Geometry check sheet. Reference: drawing and pictorial views, mm from the part's lowest x, y, z. A direction names the side the tool comes from. Round coordinates to 2 decimals unless told otherwise and drop trailing zeros. Order: outer loops, then holes, each group sorted by start corner. A loop starts at its lowest first (then second) coordinate and runs counter-clockwise, first axis right, second up. Notation, with made-up numbers: (37, 51.25) -> (70, 51.25) arc R28 cw to (70, 72.25) -> close; hole circle Ø8 at (-33, 76.25). An arc over 180 degrees is marked (long way). Put each result on its own line as item: value.
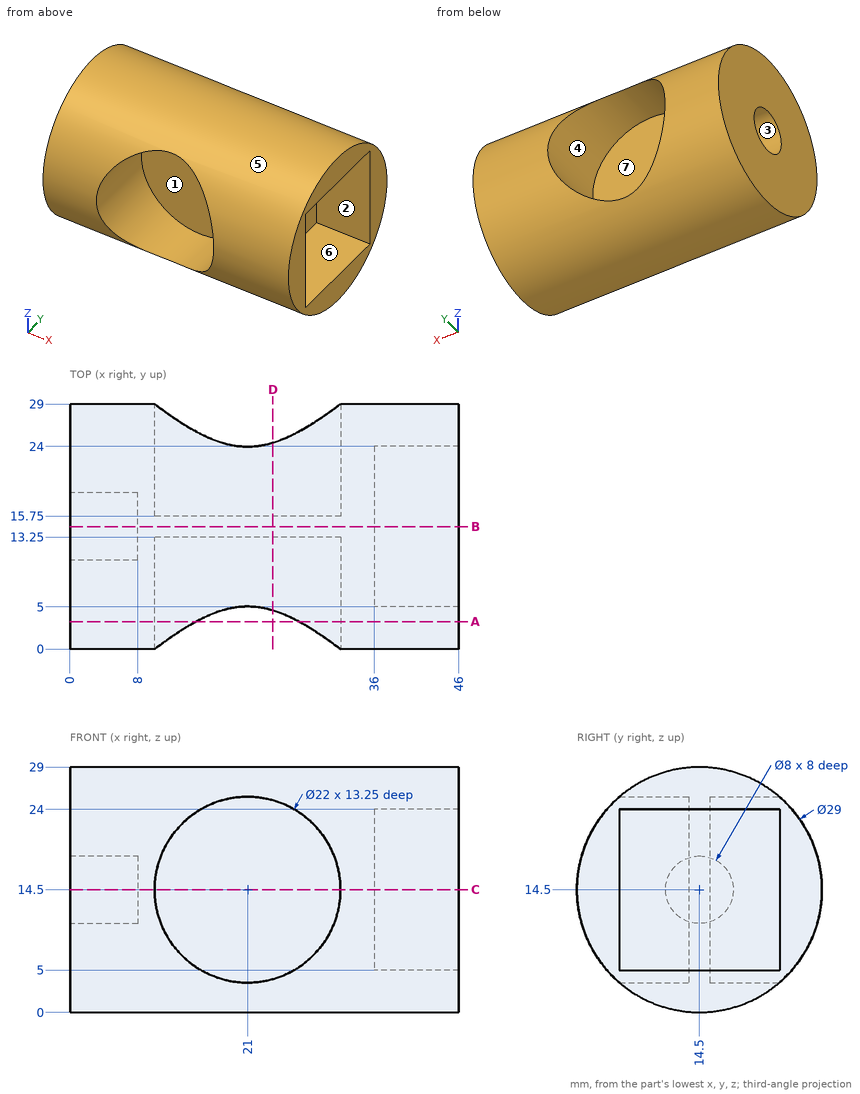
Item 1: Sectioned sample at B-B, the plane y = 14.5. Record the boundary of the cut face in (x, z).
Geometry check:
outline: (0, 0) -> (46, 0) -> (46, 5) -> (36, 5) -> (36, 24) -> (46, 24) -> (46, 29) -> (0, 29) -> (0, 18.5) -> (8, 18.5) -> (8, 10.5) -> (0, 10.5) -> close
Item 2: Sectioned sample at A-A, the plane y = 3.25. Record the boundary of the cut face in (x, z).
Geometry check:
outline: (0, 5.35) -> (14.89, 5.35) arc R11 cw to (14.89, 23.65) -> (0, 23.65) -> close; (27.11, 5.35) -> (46, 5.35) -> (46, 23.65) -> (27.11, 23.65) arc R11 cw to start
Item 3: Material ranges on line 1 along Y through (x, z) = (2.25, 14.5); line 2 along Y through (x, z) = (21, 22.75); line 3 along Z through (x, y) = (15, 14), recorded low to high.
Geometry check:
line 1: 0 to 10.5, 18.5 to 29
line 2: 13.25 to 15.75
line 3: 0.01 to 28.99
Item 4: Depth check by flat-ended pin: pin 1 Ø3 at (x, z) = (41.5, 16.5) entering from -Y; pin 2 Ø5 at (x, y) = (38.5, 10) entering from +Z; pin 3 Ø2.5 at (y, z) = (15, 16) entering from -X. Enter the tip coordinate at first touch or a pass-through.
Geometry check:
pin 1: y = 0.01
pin 2: z = 28.86
pin 3: x = 8
Item 5: Sectioned sample at C-C, the plane z = 14.5. Record the boundary of the cut face in (x, y).
Geometry check:
outline: (0, 0) -> (10, 0) -> (10, 13.25) -> (32, 13.25) -> (32, 0) -> (46, 0) -> (46, 5) -> (36, 5) -> (36, 24) -> (46, 24) -> (46, 29) -> (32, 29) -> (32, 15.75) -> (10, 15.75) -> (10, 29) -> (0, 29) -> (0, 18.5) -> (8, 18.5) -> (8, 10.5) -> (0, 10.5) -> close
Item 6: Tool access check on the marked faces 1, 2, 3 and 4. Record the directions out of +Z, -Z, +X, -X, +Y, -Y that give a thin tool (end or side, any length) a straight path to the whole face; none if there is none.
Geometry check:
face 1: -Y
face 2: +X
face 3: -X
face 4: +Y
Item 7: Release check for a two-part mould opening along Y. For the marked faces 5, 6 and 7 record: pulls with the +Y half, pulls with the -Y half, needs draft (parallel to the pull), parting line crosses it, or undercut.
Geometry check:
face 5: parting line crosses it
face 6: undercut
face 7: pulls with the +Y half
Item 8: Sectioned sample at D-D, the plane x = 24. Record the boundary of the cut face in (y, z).
Geometry check:
outline: (4.59, 3.92) arc R14.5 ccw to (24.41, 3.92) -> (15.75, 3.92) -> (15.75, 25.08) -> (24.41, 25.08) arc R14.5 ccw to (4.59, 25.08) -> (13.25, 25.08) -> (13.25, 3.92) -> close
